from build123d import *

# Parameters (mm, degrees)
F1_DEPTH     = 38.1
F2_SIZE      = 22.86
F3_W         = 104.742500931
F3_H         = 73.319750838
F4_DEPTH     = 38.1
F5_T1_DEPTH  = 93.1636902777
F5_T3_DEPTH  = 93.1636902777
F5_T5_DEPTH  = 93.1636902777
F5_T7_DEPTH  = 93.1636902777
F5_T9_DEPTH  = 93.1636902777
F5_T11_DEPTH = 93.1636902777


# Not quite as in the source:
# - a fillet or chamfer that OpenCascade refuses, or shapes differently, is made with other operations: its cross-section is extruded or revolved along the edge and cut away or added


with BuildPart() as f1:
    # F0 (on Top) → F1 (new body, symmetric)
    with BuildSketch(Plane.XY):
        Polygon((15.5198623998, 23.1162996964), (-12.2593715787, 24.9987449497), (-27.7792339785, 1.8824452533), (-15.5198623998, -23.1162996964), (12.2593715787, -24.9987449497), (27.7792339785, -1.8824452533), align=None)
    extrude(amount=F1_DEPTH, both=True)

    # F2
    f2_edges = [f1.edges().sort_by_distance(p)[0] for p in [
        (21.649548, 10.616927, 38.1),
        (1.630245, 24.057522, 38.1),
        (-20.019303, 13.440595, 38.1),
        (-21.649548, -10.616927, 38.1),
        (-1.630245, -24.057522, 38.1),
        (20.019303, -13.440595, 38.1),
    ]]
    chamfer(f2_edges, length=F2_SIZE)

    # F3 (on Right) → F4 (cut, symmetric)
    with BuildSketch(Plane.YZ):
        with Locations((-5.571493879, -24.6362821199)):
            Rectangle(F3_W, F3_H)
    extrude(amount=F4_DEPTH, both=True, mode=Mode.SUBTRACT)

    # F5: chamfer of 12.7 on 6 edges, made by hand

    # F5_s2 → F5_t1 (cut)
    with BuildSketch(Plane(origin=(-20.5101939484, 41.8234412828, 0), x_dir=(0, 0, 1), z_dir=(0.4403044553, -0.8978485322, 0))):
        Polygon((24.7235932991, -24.1126954201), (12.0235932991, -11.4126954201), (12.0235932991, -24.1126954201), align=None)
    extrude(amount=F5_T1_DEPTH, mode=Mode.SUBTRACT)

    # F5_s4 → F5_t3 (cut)
    with BuildSketch(Plane(origin=(25.9650656504, 38.6740696373, 0), x_dir=(0, 0, 1), z_dir=(-0.55740741, -0.8302391097, 0))):
        Polygon((12.0235932991, -11.4126954201), (24.7235932991, -24.1126954201), (12.0235932991, -24.1126954201), align=None)
    extrude(amount=F5_T3_DEPTH, mode=Mode.SUBTRACT)

    # F5_s6 → F5_t5 (cut)
    with BuildSketch(Plane(origin=(46.4752595988, -3.1493716455, 0), x_dir=(0, 0, 1), z_dir=(-0.9977118652, 0.0676094224, 0))):
        Polygon((12.0235932991, -11.4126954201), (24.7235932991, -24.1126954201), (12.0235932991, -24.1126954201), align=None)
    extrude(amount=F5_T5_DEPTH, mode=Mode.SUBTRACT)

    # F5_s8 → F5_t7 (cut)
    with BuildSketch(Plane(origin=(20.5101939484, -41.8234412828, 0), x_dir=(0, 0, 1), z_dir=(-0.4403044553, 0.8978485322, 0))):
        Polygon((12.0235932991, -11.4126954201), (24.7235932991, -24.1126954201), (12.0235932991, -24.1126954201), align=None)
    extrude(amount=F5_T7_DEPTH, mode=Mode.SUBTRACT)

    # F5_s10 → F5_t9 (cut)
    with BuildSketch(Plane(origin=(-25.9650656504, -38.6740696373, 0), x_dir=(0, 0, 1), z_dir=(0.55740741, 0.8302391097, 0))):
        Polygon((12.0235932991, -11.4126954201), (24.7235932991, -24.1126954201), (12.0235932991, -24.1126954201), align=None)
    extrude(amount=F5_T9_DEPTH, mode=Mode.SUBTRACT)

    # F5_s12 → F5_t11 (cut)
    with BuildSketch(Plane(origin=(-46.4752595988, 3.1493716455, 0), x_dir=(0, 0, 1), z_dir=(0.9977118652, -0.0676094224, 0))):
        Polygon((12.0235932991, -11.4126954201), (24.7235932991, -24.1126954201), (12.0235932991, -24.1126954201), align=None)
    extrude(amount=F5_T11_DEPTH, mode=Mode.SUBTRACT)


solid = f1.part
Design review of the part built by this model. Coordinates are the model's own, in mm. Give positions to 0.01 mm unless a question says otherwise; leave off trailing zeros. Write each loop counter-clockwise with the first axis right and the second up, starting at its lowest first coordinate (ties: lowest second). Pieces come first, ordered by that corner, then holes. Notation, with made-up numbers: M 52.25,-31.5 L 76.25,-31.5 A25 cw 76.25,-1.5 Z; hole C 27,86 d5. An arc over 180 degrees is marked long. Answer as a JSON object with one key per item and string values. Group by question number.
1) We need section C-C (y = -5.5). Give the boundary of the cut face in (x, z), and give its area (3 significant figures).
2) We need section D-D (x = 11.5). Give the boundary of the cut face in (y, z).
3) For line 1 along Z through (x, y) = (2, 11); line 2 along Y through (x, z) = (-12.5, 14.75); line 3 along Y through (x, z) = (13, 27), list the stretches that pass through material, from the lowest coordinate up.
4) Clearance check with flat-ended pins moving along their axes: pin 1 Ø8 at (y, z) = (8.5, 25) entering from +X; pin 2 Ø6 at (x, y) = (15.5, 1.5) entering from +Z; pin 3 Ø3 at (x, y) = (9.5, -7) entering from +Z. State where each tip first meets the part, or that it passes through.
5) We need section B-B (z = 17.75). Give the boundary of the cut face in (x, y), and give its area (3 significant figures).
6) We need section A-A (x = 6.5). Give the boundary of the cut face in (y, z), and give its area (3 significant figures).
Answer key:
{
 "1": {"outline": "M -18.88,19.98 L -10.01,12.02 L 10.05,12.02 L 19.64,19.98 L 2.7,34.05 L -3.69,33.62 Z", "area": "544 mm²"},
 "2": {"outline": "M -17.62,19.98 L -3.35,12.02 L 2.47,12.02 L 17.13,18.48 L 18.64,19.98 L 17.13,21.49 L -0.78,29.37 Z"},
 "3": {"line 1": "z = 12.02 to 28.24", "line 2": "y = -6.62 to 6.75", "line 3": "y = -2.8 to 1.55"},
 "4": {"pin 1": "stops at x = 16.69", "pin 2": "stops at z = 27.78", "pin 3": "stops at z = 29.06"},
 "5": {"outline": "M -19.75,1.34 L -11.03,-16.43 L 8.71,-17.77 L 19.75,-1.34 L 11.03,16.43 L -8.71,17.77 Z", "area": "1,020 mm²"},
 "6": {"outline": "M -19.86,19.98 L -13.25,13.4 L -10.79,12.02 L 11,12.02 L 18.97,19.98 L 9.68,29.25 L -0.44,33.71 L -13.25,26.57 Z", "area": "556 mm²"}
}
